Design review of the part built by this model. Coordinates are the model's own, in mm. Face numbers are marked on the shaded views. A direction names the side the tool comes from. Coordinates: 2 decimals unless noted, no trailing zeros. Write each loop counter-clockwise with the first axis right and the second up, starting at its lowest first coordinate (ties: lowest second). Pieces come first, ordered by that corner, then holes. Notation, with made-up numbers: (14.5, 60) -> (52.5, 60) arc R17 ccw to (52.5, 69) -> close; hole circle Ø6 at (-4, 89.5). An arc over 180 degrees is marked (long way). Answer in a Markdown table with one row per item. Add a question column.
Item 1: Take a section at D-D, the plane z = 5. Write out the cut boundary in (x, y).
Item 2: Take a section at C-C, the plane x = -17.5. Write out the cut boundary in (y, z).
Item 3: Draft analysis for pull direction X (two halves, no side actions). For the marked faces 1, 2, 3 and 4, state which applies: released by +X, released by -X, zero draft, split by the parting line, or undercut.
Item 4: Take a section at B-B, the plane y = -23. Write out the cut boundary in (x, z).
Item 5: Clearance check with flat-ended pins moving along their axes: P1, Ø2, axis at x = -9, y = -14.5, coming from the -Z side (3 decimals); P2, Ø6.5, axis at x = 2.5, y = -22.5, coming from the +Z side; P3, Ø4, axis at y = -22, z = 2, coming from the -X side; P4, Ø2, axis at y = -18.5, z = -11.5, coming from the -X side. State where each tip first meets the part, or that it passes through.
Item 6: To check wall thickness, follow line 1 (Z direction, x = -1, y = -22); line 2 (Z direction, x = 7.5, y = -4); line 3 (X direction, y = -17.5, z = 2.5). State the ranges of each line that lie inside material, in increasing order.
Item 7: For the marked faces 5, 6, 7 and 8, list the 3-axis set-ups (+Z, -Z, +X, -X, +Y, -Y) from which the entire face can be reached by the end or side of a thin tool; tool diameter is ignored.
Item 8: Take a section at A-A, the plane x = 0. Write out the cut boundary in (y, z).
Solid Edge part; units mm, degrees
sketch "Sketch1" plane through (0, 0, 0) normal (0, -1, 0) x (1, 0, 0)
  line L0 (18.5, -18.5) -> (18.5, 18.5)
  line L1 (18.5, 18.5) -> (-18.5, 18.5)
  line L2 (-18.5, 18.5) -> (-18.5, -18.5)
  line L3 (-18.5, -18.5) -> (18.5, -18.5)
extrude "Protrusion1" add sketch "Sketch1" along normal blind 18
sketch "Sketch2" plane through (18.5, -9, 0) normal (1, 0, 0) x (0, 0, 1)
  line L0 (-9, 9) -> (-18.5, 9)
  line L1 (-18.5, 9) -> (-18.5, -9)
  line L2 (-18.5, -9) -> (-9, 9)
  line L3 (9, 9) -> (18.5, -9)
  line L4 (18.5, -9) -> (18.5, 9)
  line L5 (18.5, 9) -> (9, 9)
extrude "ExtrudedCutout_5" cut sketch "Sketch2" against normal blind 37 and the other way blind 1
extrude "ExtrudedCutout_6" [suppressed]
sketch "Sketch3" plane through (0, -9, 26) normal (0, 0, 1) x (-1, 0, 0)
  line L0 (-9, 9) -> (-18.5, -9)
  line L1 (-18.5, -9) -> (-26, -9)
  line L2 (-26, -9) -> (-26, 9)
  line L3 (-26, 9) -> (-9, 9)
  line L4 (9, 9) -> (26, 9)
  line L5 (26, 9) -> (26, -9)
  line L6 (26, -9) -> (18.5, -9)
  line L7 (18.5, -9) -> (9, 9)
extrude "ExtrudedCutout_7" cut sketch "Sketch3" against normal blind 52 and the other way blind 1
sketch "Sketch4" plane through (0, 0, 0) normal (0, -1, 0) x (1, 0, 0)
  line L0 (26, 26) -> (-26, 26)
  line L1 (-26, 26) -> (-26, -26)
  line L2 (-26, -26) -> (26, -26)
  line L3 (26, -26) -> (26, 26)
extrude "ExtrudedProtrusion_7" add sketch "Sketch4" against normal blind 5
sketch "Sketch5" plane through (0, -18, 0) normal (0, -1, 0) x (-1, 0, 0)
  line L0 (9, -9) -> (-9, -9)
  line L1 (-9, -9) -> (-9, 9)
  line L2 (-9, 9) -> (9, 9)
  line L3 (9, 9) -> (9, -9)
extrude "ExtrudedProtrusion_8" add sketch "Sketch5" along normal blind 8
shell "Thinwall1" thickness 5 removed faces 2 at (-16.8133, 5, 17.8533) at (-5.82, -26, -6.18)
shell "Thinwall2" [suppressed]
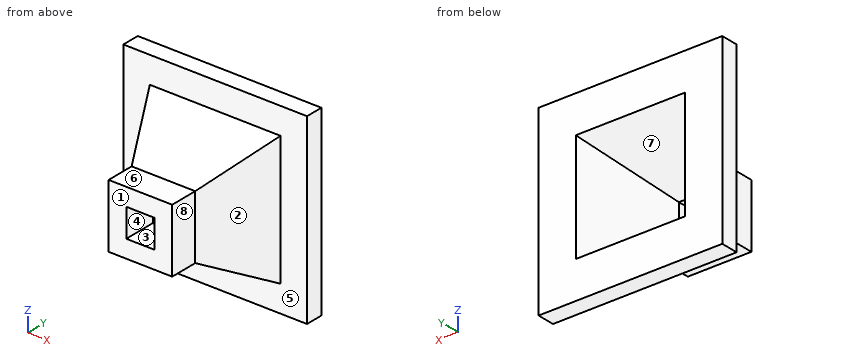
Answers:
| question | item | result |
|---|---|---|
| 1 | outline | (-26, 0) -> (-18.5, 0) -> (-9, -18) -> (-9, -26) -> (9, -26) -> (9, -18) -> (18.5, 0) -> (26, 0) -> (26, 5) -> (15.49, 5) -> (5, -14.87) -> (-5, -14.87) -> (-15.49, 5) -> (-26, 5) -> close |
| 2 | outline | (-1.89, -17.5) -> (0, -18.5) -> (0, -26) -> (5, -26) -> (5, 26) -> (0, 26) -> (0, 18.5) -> (-1.89, 17.5) -> close |
| 3 | face 1 | zero draft |
| 3 | face 2 | released by +X |
| 3 | face 3 | undercut |
| 3 | face 4 | undercut |
| 4 | outline | (-9, -9) -> (9, -9) -> (9, 9) -> (-9, 9) -> close; hole (-4, -4) -> (4, -4) -> (4, 4) -> (-4, 4) -> close |
| 5 | P1 | stops at z = -11.375 |
| 5 | P2 | stops at z = 9 |
| 5 | P3 | stops at x = -9 |
| 5 | P4 | passes through |
| 6 | line 1 | z = -9 to -4, 4 to 9 |
| 6 | line 2 | z = -16.39 to -10.74, 10.74 to 16.39 |
| 6 | line 3 | x = -9.26 to -4, 4 to 9.26 |
| 7 | face 5 | -Y |
| 7 | face 6 | +Z, +X, -X, -Y |
| 7 | face 7 | +Y |
| 7 | face 8 | +Z, -Z, +X, -Y |
| 8 | outline | (-26, -9) -> (-18, -9) -> (0, -18.5) -> (0, -26) -> (5, -26) -> (5, -15.49) -> (-16.76, -4) -> (-26, -4) -> close; (-26, 4) -> (-16.76, 4) -> (5, 15.49) -> (5, 26) -> (0, 26) -> (0, 18.5) -> (-18, 9) -> (-26, 9) -> close |
